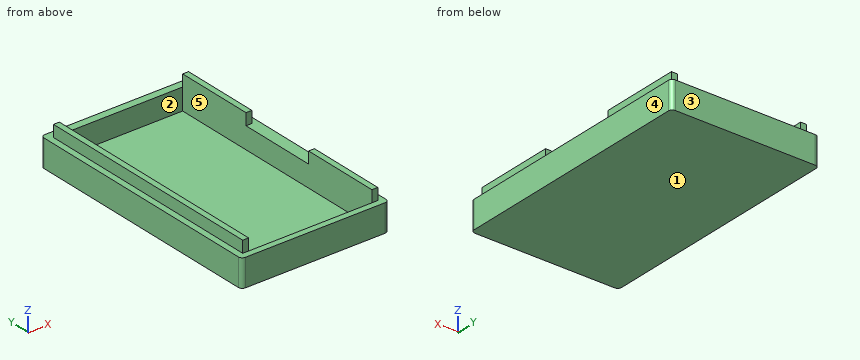
from build123d import *

# Parameters (mm, degrees)
F0_W     = 37.693575
F0_H     = 64.1
F0_W_2   = 31.5
F0_H_2   = 60.5
F1_DEPTH = 7
F2_DEPTH = 1.5
F3_W     = 1.5
F3_H     = 60.5
F4_DEPTH = 3
F5_R     = 1
F6_W     = 20
F6_H     = 3
F7_DEPTH = 1.5


with BuildPart() as f1:
    # F0 (on Top) → F1 (new body)
    with BuildSketch(Plane.XY):
        with Locations((0.003213, 0.2)):
            Rectangle(F0_W, F0_H)
        Rectangle(F0_W_2, F0_H_2, mode=Mode.SUBTRACT)
    extrude(amount=F1_DEPTH)

    # F0 (on Top) → F2 (join)
    with BuildSketch(Plane.XY):
        Rectangle(F0_W_2, F0_H_2)
    extrude(amount=F2_DEPTH)

    # F3 (on face) → F4 (join)
    with BuildSketch(Plane.XY.offset(7)):
        with Locations((-16.5, 0)):
            Rectangle(F3_W, F3_H)
        with Locations((16.5, 0)):
            Rectangle(F3_W, F3_H)
    extrude(amount=F4_DEPTH)

    # F5
    f5_edges = [f1.edges().sort_by_distance(p)[0] for p in [
        (-18.843575, -31.85, 3.5),
        (18.85, -31.85, 3.5),
        (18.85, 32.25, 3.5),
        (-18.843575, 32.25, 3.5),
    ]]
    fillet(f5_edges, radius=F5_R)

    # F6 (on face) → F7 (cut, through all)
    with BuildSketch(Plane.YZ.offset(17.25)):
        with Locations((0, 8.5)):
            Rectangle(F6_W, F6_H)
    extrude(amount=-F7_DEPTH, mode=Mode.SUBTRACT)


solid = f1.part
Can you work these out from the model? Positions are in its coordinate system, mm. Face numbers are marked on the shaded views. A direction names the side the tool comes from. Coordinates: 2 decimals unless noted, no trailing zeros. Order: outer loops, then holes, each group sorted by start corner. A loop starts at its lowest first (then second) coordinate and runs counter-clockwise, first axis right, second up. Notation, with made-up numbers: (-30.75, 24) - (21.25, 24) arc R23 ccw to (21.25, 43) - close; hole circle Ø5 at (67.25, 11.5). An arc over 180 degrees is marked (long way). Answer as a JSON object with one key per item and string values. Group by question number.
Q1. Imagine slicing it at C-C (z = 4). Please give me the cut outline in (x, y), and give its area (3 significant figures).
Q2. I need wall thicknesses on line 1 (X direction, y = 21, z = 6.5); line 2 (Y direction, x = -12, z = 5.5); line 3 (X direction, y = -22, z = 7.5). Which ranges of each line are inside material? Lowest first, please. Write a range as from..to.
Q3. On a 3-axis mill with a long thin cutter (end or side, diameter ignored), from which of +Z, -Z, +X, -X, +Y, -Y can I reach the whole of each face in a straight line? I mean the marked faces 1 and 2. Say none if no direction works.
Q4. Imagine slicing it at B-B (x = 2). Please give me the cut outline in (y, z).
Q5. Will these pins go through, and if not, where does the flat tip stop? P1, Ø9.5, axis at x = 3, y = -13, coming from the +Z side; P2, Ø1.2, axis at x = 16.5, z = 9, coming from the +Y side; P3, Ø1.5, axis at y = -2.5, z = 8.5, coming from the -X side.
Q6. We'd pull the mould along X, two halves only. Please class the marked faces 3, 4 and 5: +X half, -X half, draft (parallel to the pull), parting line (faces both ways), or undercut.
Q7. Imagine slicing it at D-D (y = -3). Please give me the cut outline in (x, z).
Q8. Imagine slicing it at A-A (z = 8.5). Please give me the cut outline in (x, y).
Determined:
{
 "1": {"outline": "(-18.84, -30.85) arc R1 ccw to (-17.84, -31.85) - (17.85, -31.85) arc R1 ccw to (18.85, -30.85) - (18.85, 31.25) arc R1 ccw to (17.85, 32.25) - (-17.84, 32.25) arc R1 ccw to (-18.84, 31.25) - close; hole (-15.75, -30.25) - (15.75, -30.25) - (15.75, 30.25) - (-15.75, 30.25) - close", "area": "510 mm2"},
 "2": {"line 1": "x = -18.84..-15.75, 15.75..18.85", "line 2": "y = -31.85..-30.25, 30.25..32.25", "line 3": "x = -17.25..-15.75, 15.75..17.25"},
 "3": {"face 1": "-Z, +X, -X, +Y, -Y", "face 2": "+Z"},
 "4": {"outline": "(-31.85, 0) - (32.25, 0) - (32.25, 7) - (30.25, 7) - (30.25, 1.5) - (-30.25, 1.5) - (-30.25, 7) - (-31.85, 7) - close"},
 "5": {"P1": "stops at z = 1.5", "P2": "stops at y = 30.25", "P3": "stops at x = -17.25"},
 "6": {"face 3": "draft", "face 4": "+X half", "face 5": "undercut"},
 "7": {"outline": "(-18.84, 0) - (18.85, 0) - (18.85, 7) - (15.75, 7) - (15.75, 1.5) - (-15.75, 1.5) - (-15.75, 10) - (-17.25, 10) - (-17.25, 7) - (-18.84, 7) - close"},
 "8": {"outline": "(-17.25, -30.25) - (-15.75, -30.25) - (-15.75, 30.25) - (-17.25, 30.25) - close; (15.75, -30.25) - (17.25, -30.25) - (17.25, -10) - (15.75, -10) - close; (15.75, 10) - (17.25, 10) - (17.25, 30.25) - (15.75, 30.25) - close"}
}
